```python
from build123d import *

# Parameters (mm, degrees)
BASE_FLANGE1_DEPTH            = 38.1
SKETCH4_W                     = 50.8
SKETCH4_H                     = 17.78
TAB1_DEPTH                    = 1.5875
SKETCH5_W                     = 50.8
SKETCH5_H                     = 17.78
TAB2_DEPTH                    = 1.5875
EDGE_FLANGE4_STRIP_W          = 7.8232
EDGE_FLANGE4_STRIP_H          = 1.5875
EDGE_FLANGE4_STRIP_CUT_DEPTH  = 38.1
EDGE_FLANGE4_RELIEF_W         = 8.61695
EDGE_FLANGE4_RELIEF_H         = 0.79375
EDGE_FLANGE4_RELIEF_CUT_DEPTH = 1.5875
EDGE_FLANGE4_DEPTH            = 38.1
SKETCH18_R                    = 14.351
CUT_EXTRUDE1_DEPTH            = 110.605811015
SKETCH19_W                    = 38.1
SKETCH19_H                    = 25.4
TAB3_DEPTH                    = 1.5875
SKETCH20_W                    = 38.1
SKETCH20_H                    = 25.4
TAB4_DEPTH                    = 1.5875
SKETCH21_R                    = 2.54
CUT_EXTRUDE2_DEPTH            = 117.856930597
CUT_EXTRUDE4_DEPTH            = 97.862741461


# Sheet-metal steps are written as plain solids
with BuildPart() as part:
    # Sketch1 → Base-Flange1 (new, symmetric)
    with BuildSketch(Plane.XY):
        with BuildLine():
            Line((5.148952002, 26.77051137), (28.224852002, 26.77051137))
            ThreePointArc((28.224852002, 26.77051137), (29.868238872, 26.08979824), (30.548952002, 24.44641137))
            Line((30.548952002, 24.44641137), (30.548952002, -7.41788863))
            ThreePointArc((30.548952002, -7.41788863), (29.868238872, -9.061275501), (28.224852002, -9.74198863))
            Line((28.224852002, -9.74198863), (-32.951047998, -9.74198863))
            Line((-32.951047998, -9.74198863), (-32.951047998, -8.15448863))
            Line((-32.951047998, -8.15448863), (28.224852002, -8.15448863))
            ThreePointArc((28.224852002, -8.15448863), (28.745706857, -7.938743485), (28.961452002, -7.41788863))
            Line((28.961452002, -7.41788863), (28.961452002, 24.44641137))
            ThreePointArc((28.961452002, 24.44641137), (28.745706857, 24.967266225), (28.224852002, 25.18301137))
            Line((28.224852002, 25.18301137), (5.148952002, 25.18301137))
            Line((5.148952002, 25.18301137), (5.148952002, 26.77051137))
        make_face()
    extrude(amount=BASE_FLANGE1_DEPTH, both=True)

    # Sketch4 → Tab1 (add)
    with BuildSketch(Plane(origin=(0, 26.77051137, 0), x_dir=(1, 0, 0), z_dir=(0, 1, 0))):
        with Locations((-20.251047998, -29.21)):
            Rectangle(SKETCH4_W, SKETCH4_H)
    extrude(amount=-TAB1_DEPTH)

    # Sketch5 → Tab2 (add)
    with BuildSketch(Plane(origin=(0, 26.77051137, 0), x_dir=(1, 0, 0), z_dir=(0, 1, 0))):
        with Locations((-20.251047998, 29.21)):
            Rectangle(SKETCH5_W, SKETCH5_H)
    extrude(amount=-TAB2_DEPTH)

    # Edge-Flange4 strip (across the edge) → Edge-Flange4 strip cut (cut)
    with BuildSketch(Plane(origin=(5.148952002, 26.77051137, -19.05), x_dir=(1, 0, 0), z_dir=(0, 0, 1))):
        with Locations((-3.175, -0.79375)):
            Rectangle(EDGE_FLANGE4_STRIP_W, EDGE_FLANGE4_STRIP_H)
    extrude(amount=EDGE_FLANGE4_STRIP_CUT_DEPTH, mode=Mode.SUBTRACT)

    # Edge-Flange4 relief (on the sheet) → Edge-Flange4 relief cut (cut)
    with BuildSketch(Plane(origin=(5.885552002, 26.77051137, -19.05), x_dir=(1, 0, 0), z_dir=(0, 1, 0))):
        with Locations((-3.514725, 0.396875)):
            Rectangle(EDGE_FLANGE4_RELIEF_W, EDGE_FLANGE4_RELIEF_H)
        with Locations((-3.514725, -38.496875)):
            Rectangle(EDGE_FLANGE4_RELIEF_W, EDGE_FLANGE4_RELIEF_H)
    extrude(amount=-EDGE_FLANGE4_RELIEF_CUT_DEPTH, mode=Mode.SUBTRACT)

    # Edge-Flange4 section (across the edge) → Edge-Flange4 (add)
    with BuildSketch(Plane(origin=(5.148952002, 26.77051137, -19.05), x_dir=(1, 0, 0), z_dir=(0, 0, 1))):
        with BuildLine():
            Line((-1.5875, 0.7366), (-1.5875, 57.15))
            Line((-1.5875, 57.15), (0, 57.15))
            Line((0, 57.15), (0, 0.7366))
            ThreePointArc((0, 0.7366), (0.215745145, 0.215745145), (0.7366, 0))
            Line((0.7366, 0), (0.7366, -1.5875))
            ThreePointArc((0.7366, -1.5875), (-0.90678687, -0.90678687), (-1.5875, 0.7366))
        make_face()
    extrude(amount=EDGE_FLANGE4_DEPTH)

    # Sketch18 → Cut-Extrude1 (cut, through all)
    with BuildSketch(Plane(origin=(0, -8.15448863, 0), x_dir=(1, 0, 0), z_dir=(0, 1, 0))):
        with Locations(Location((-15.488547998, 0, 0), (0, 0, 180))):
            Circle(SKETCH18_R)
    extrude(amount=-CUT_EXTRUDE1_DEPTH, mode=Mode.SUBTRACT)

    # Sketch19 → Tab3 (add)
    with BuildSketch(Plane(origin=(0, 26.77051137, 0), x_dir=(1, 0, 0), z_dir=(0, 1, 0))):
        with Locations((-26.601047998, -50.8)):
            Rectangle(SKETCH19_W, SKETCH19_H)
    extrude(amount=-TAB3_DEPTH)

    # Sketch20 → Tab4 (add)
    with BuildSketch(Plane(origin=(0, 26.77051137, 0), x_dir=(1, 0, 0), z_dir=(0, 1, 0))):
        with Locations((-26.601047998, 50.8)):
            Rectangle(SKETCH20_W, SKETCH20_H)
    extrude(amount=-TAB4_DEPTH)

    # Sketch21 → Cut-Extrude2 (cut, through all)
    with BuildSketch(Plane(origin=(5.148952002, 0, 0), x_dir=(0, 0, -1), z_dir=(1, 0, 0))):
        with Locations(Location((-9.525, 32.86651137, 0), (0, 0, 90))):
            Circle(SKETCH21_R)
        with Locations(Location((9.525, 32.86651137, 0), (0, 0, 90))):
            Circle(SKETCH21_R)
        with Locations(Location((-9.525, 79.85651137, 0), (0, 0, 90))):
            Circle(SKETCH21_R)
        with Locations(Location((9.525, 79.85651137, 0), (0, 0, 90))):
            Circle(SKETCH21_R)
    extrude(amount=-CUT_EXTRUDE2_DEPTH, mode=Mode.SUBTRACT)

    # Sketch24 → Cut-Extrude4 (cut, through all)
    with BuildSketch(Plane(origin=(0, 26.77051137, 0), x_dir=(1, 0, 0), z_dir=(0, 1, 0))):
        with BuildLine():
            Line((-39.301047998, -48.26), (-15.19816231, -48.26))
            ThreePointArc((-15.19816231, -48.26), (-12.65816231, -50.8), (-15.19816231, -53.34))
            Line((-15.19816231, -53.34), (-39.301047998, -53.34))
            ThreePointArc((-39.301047998, -53.34), (-41.841047998, -50.8), (-39.301047998, -48.26))
        make_face()
    cut_extrude4 = extrude(amount=-CUT_EXTRUDE4_DEPTH, mode=Mode.SUBTRACT)

    # Mirror1: Cut-Extrude4 across plane
    add(cut_extrude4.mirror(Plane.XY), mode=Mode.SUBTRACT)


solid = part.part
```
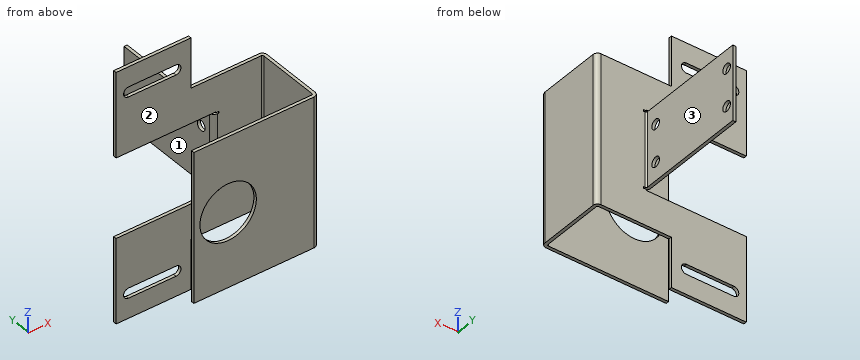
Input: part model. Units: mm. Frame: model coordinates. Face numbers are marked on the shaded views. A direction names the side the tool comes from. Give positions to 0.01 mm unless a question says otherwise; leave off trailing zeros. Loops run counter-clockwise (first coordinate to the right, second up) from the corner with the lowest first, then second, coordinate; pieces in that order, holes last.
1) Reachability of the marked faces 1, 2 and 3 from +Z, -Z, +X, -X, +Y, -Y: full face, straight path, thin tool, end or side. Return the list, or none.
A:
face 1: +Z, -Z, -X, +Y
face 2: +Z, -Z, -X
face 3: +Z, -Z, +X, +Y
2) Section query D-D on y = 33.5. Return the cut outline in (x, z).
A:
outline: (3.56, -19.05) - (5.15, -19.05) - (5.15, -11.98) - (3.56, -11.98) - close; (3.56, -7.07) - (5.15, -7.07) - (5.15, 7.07) - (3.56, 7.07) - close; (3.56, 11.98) - (5.15, 11.98) - (5.15, 19.05) - (3.56, 19.05) - close
3) Line query: L1, parallel to Y at x = 22, z = -23.5; L2, parallel to Y at x = -25, z = -57.5; L3, parallel to X at y = 22, z = 13.5. Output: solid intervals per line, ascending.
A:
L1: y = -9.74 to -8.15, 25.18 to 26.77
L2: y = 25.18 to 26.77
L3: x = 28.96 to 30.55
4) Section query A-A on x = 12.5. Return the cut outline in (y, z).
A:
outline: (-9.74, -38.1) - (-8.15, -38.1) - (-8.15, 38.1) - (-9.74, 38.1) - close; (25.18, -38.1) - (26.77, -38.1) - (26.77, 38.1) - (25.18, 38.1) - close
5) Contact query for flat-ended pins moving along their axis: pin 1 (1.3 mm diameter, centred on y = -8.5, z = 8, fed in from -X); pin 2 (2.5 mm diameter, centred on x = 5.5, y = 51, fed in from -Z); pin 3 (0.6 mm diameter, centred on y = 26, z = 19.5, fed in from -X); pin 4 (1.5 mm diameter, centred on x = -5, z = -41, fed in from +Y). Output: stop coordinate, or through.
A:
pin 1: stops at x = -32.95
pin 2: stops at z = -19.05
pin 3: stops at x = 6.68
pin 4: passes through
6) Section query C-C on x = -10.5. Return the cut outline in (y, z), and give its area (3 significant figures).
A:
outline: (-9.74, -38.1) - (-8.15, -38.1) - (-8.15, -13.46) - (-9.74, -13.46) - close; (-9.74, 13.46) - (-8.15, 13.46) - (-8.15, 38.1) - (-9.74, 38.1) - close; (25.18, -63.5) - (26.77, -63.5) - (26.77, -20.32) - (25.18, -20.32) - close; (25.18, 20.32) - (26.77, 20.32) - (26.77, 63.5) - (25.18, 63.5) - close
area: 215 mm2
7) Section query B-B on z = 0. Return the cut outline in (x, y), and give its area (3 significant figures).
A:
outline: (-32.95, -9.74) - (-29.84, -9.74) - (-29.84, -8.15) - (-32.95, -8.15) - close; (-1.14, -9.74) - (28.22, -9.74) arc R2.32 ccw to (30.55, -7.42) - (30.55, 24.45) arc R2.32 ccw to (28.22, 26.77) - (5.89, 26.77) arc R0.74 cw to (5.15, 27.51) - (5.15, 83.92) - (3.56, 83.92) - (3.56, 27.51) arc R2.32 ccw to (5.89, 25.18) - (28.22, 25.18) arc R0.74 cw to (28.96, 24.45) - (28.96, -7.42) arc R0.74 cw to (28.22, -8.15) - (-1.14, -8.15) - close
area: 239 mm2
